Part model, mm, in its own coordinate system. Give positions to 0.01 mm unless a question says otherwise; leave off trailing zeros. Write each loop counter-clockwise with the first axis right and the second up, starting at its lowest first coordinate (ties: lowest second). Pieces come first, ordered by that corner, then holes. Notation, with made-up numbers: M 20.5,13.5 L 29.5,13.5 A27 cw 29.5,32.5 Z; hole C 60,-0.5 d9. An arc over 180 degrees is marked long. Write item = value, one per line. Start each with the question number.
from build123d import *

# Parameters (mm, degrees)
SKETCH1_W           = 6.35
SKETCH1_H           = 71.247
BOSS_EXTRUDE1_DEPTH = 2.9972


with BuildPart() as part:
    # Sketch1 → Boss-Extrude1 (new body)
    with BuildSketch(Plane.XY):
        Polygon((0, 107.95), (-146.05, 107.95), (-146.05, 95.25), (-139.7, 95.25), (-139.7, 24.003), (-139.7, -107.95), (0, -107.95), align=None)
        with Locations((-142.875, 59.6265)):
            Rectangle(SKETCH1_W, SKETCH1_H)
        Polygon((146.05, 107.95), (0, 107.95), (0, -107.95), (139.7, -107.95), (139.7, 24.003), (139.7, 95.25), (146.05, 95.25), align=None)
        with Locations((142.875, 59.6265)):
            Rectangle(SKETCH1_W, SKETCH1_H)
    extrude(amount=BOSS_EXTRUDE1_DEPTH)


solid = part.part
Q1. Probe line 1 along X through (y, z) = (1.5, 1.55). List the from-to ranges inside material, lowest first.
Q2. Slice it at B-B (y = -77). Give the cut face in (x, z), and give its area (3 significant figures).
Q3. Slice it at A-A (z = 0.7). Give the cut face in (x, y).
Q4. Two-plate mould, pull along Z, no slides. Class faces 1 (the face through (-2, 2, 2.997)), 2 (the face through (-2, 2, 0)): +Z half, -Z half, draft (parallel to the pull), parting line (faces both ways), or undercut.
Q5. Drop flat-ended pins along their axis: P1, Ø1.5, axis at y = -8, z = 1, coming from the +X side; P2, Ø1.5, axis at y = -30.5, z = 1.5, coming from the -X side; P3, Ø0.9, axis at x = 142.5, z = 1.5, coming from the -Y side. Give the stop position or say it passes through.
Working result:
q1.line_1 = -139.7 to 139.7
q2.outline = M -139.7,0 L 139.7,0 L 139.7,3 L -139.7,3 Z
q2.area = 837 mm2
q3.outline = M -146.05,24 L -139.7,24 L -139.7,-107.95 L 139.7,-107.95 L 139.7,24 L 146.05,24 L 146.05,107.95 L -146.05,107.95 Z
q4.face_1 = +Z half
q4.face_2 = -Z half
q5.P1 = 139.7
q5.P2 = -139.7
q5.P3 = 24
